```python
from build123d import *

# Parameters (mm, degrees)
F1_DEPTH = 31.75
F3_DEPTH = 31.75
F4_R     = 6.111063
F5_DEPTH = 31.75
F7_DEPTH = 12.7
F9_DEPTH = 25.4


with BuildPart() as f1:
    # F0 (on Front) → F1 (new body)
    with BuildSketch(Plane.XZ):
        Polygon((-42.020088, 46.490617), (-67.420088, 46.490617), (-67.420088, 21.090617), (-3.613756, 21.090617), (-3.613756, 33.790617), (-41.713756, 33.790617), align=None)
    extrude(amount=F1_DEPTH)

    # F2 (on face) → F3 (join)
    with BuildSketch(Plane.XZ.offset(31.75)):
        with BuildLine():
            Line((-67.420088, 46.490617), (-42.020088, 46.490617))
            ThreePointArc((-42.020088, 46.490617), (-54.720088, 59.190617), (-67.420088, 46.490617))
        make_face()
    extrude(amount=-F3_DEPTH)

    # F4 (on face) → F5 (cut)
    with BuildSketch(Plane.XZ.offset(31.75)):
        with Locations((-54.720088, 46.490617)):
            Circle(F4_R)
    extrude(amount=-F5_DEPTH, mode=Mode.SUBTRACT)

    # F6 (on face) → F7 (join)
    with BuildSketch(Plane.XY.offset(33.790617)):
        with BuildLine():
            Line((-3.613756, 0), (-3.613756, -31.75))
            ThreePointArc((-3.613756, -31.75), (12.261244, -15.875), (-3.613756, 0))
        make_face()
    extrude(amount=-F7_DEPTH)

    # F8 (on face) → F9 (cut)
    with BuildSketch(Plane.XY.offset(33.790617)):
        with BuildLine():
            Line((-9.963756, -6.35), (-29.013756, -6.35))
            ThreePointArc((-29.013756, -6.35), (-35.363756, -12.7), (-29.013756, -19.05))
            Line((-29.013756, -19.05), (-9.963756, -19.05))
            ThreePointArc((-9.963756, -19.05), (-3.613756, -12.7), (-9.963756, -6.35))
        make_face()
    extrude(amount=-F9_DEPTH, mode=Mode.SUBTRACT)


solid = f1.part
```
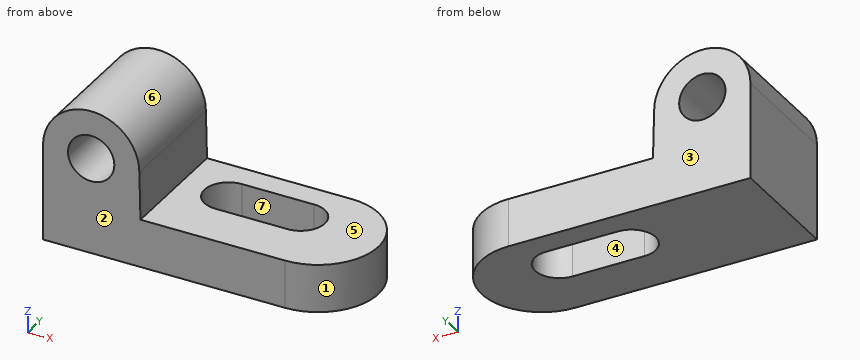
The model under review builds one solid part; all positions refer to its coordinate system, in mm. Face numbers are marked on the shaded views. A direction names the side the tool comes from. Give positions to 0.01 mm unless a question says otherwise; leave off trailing zeros. Write each loop counter-clockwise with the first axis right and the second up, starting at its lowest first coordinate (ties: lowest second). Pieces come first, ordered by that corner, then holes. Notation, with made-up numbers: M 11,-14.5 L 43,-14.5 A19 cw 43,3.5 Z; hole C 47.5,-36 d4. An arc over 180 degrees is marked long. Write item = value, one per line. Start each with the question number.
Q1. For line 1 (Z direction, x = -1.5, y = -1); line 2 (X direction, y = -7.5, z = 46.5); line 3 (Z direction, x = -51.5, y = -1), list the stretches that pass through material, from the lowest coordinate up.
Q2. Mouldability with a two-part tool opening along Y and no side actions: class the marked faces 1, 2, 3 and 4 as released by +Y, released by -Y, zero draft, split by the parting line, or undercut.
Q3. We need section B-B (z = 31.5). State the section outline as (x, y) points (3 decimals).
Q4. Machinability: for the marked faces 5, 6 and 7, which of the approach directions +Z, -Z, +X, -X, +Y, -Y give a long, thin tool a straight path to every point of the face, cutting with its end or side? Answer none if there is none.
Q5. We need section C-C (x = -57). State the section outline as (y, z) points, plus the area to 3 significant figures.
Q6. We need section D-D (y = -3). State the section outline as (x, z) points.
Q7. Clearance check with flat-ended pins moving along their axes: pin 1 (10 mm diameter, centred on x = -38, z = 49.5, fed in from +Y); pin 2 (1 mm diameter, centred on x = -42.5, y = -16.5, fed in from +Z); pin 3 (5 mm diameter, centred on x = -34.5, y = -5.5, fed in from +Z); pin 4 (4 mm diameter, centred on y = -25, z = 54, fed in from -X). State where each tip first meets the part, or that it passes through.
Q8. We need section A-A (y = -12.5). State the section outline as (x, z) points.
Result set:
q1.line_1 = 21.09 to 33.79
q1.line_2 = -67.42 to -60.83, -48.61 to -42.02
q1.line_3 = 21.09 to 41.3, 51.68 to 58.78
q2.face_1 = split by the parting line
q2.face_2 = released by -Y
q2.face_3 = released by +Y
q2.face_4 = undercut
q3.outline = M -67.42,-31.75 L -3.614,-31.75 A15.875 ccw -3.614,0 L -67.42,0 Z; hole M -29.014,-19.05 L -9.964,-19.05 A6.35 ccw -9.964,-6.35 L -29.014,-6.35 A6.35 ccw Z
q4.face_5 = +Z, +X, +Y, -Y
q4.face_6 = +Z, +Y, -Y
q4.face_7 = +Z, -Z
q5.outline = M -31.75,21.09 L 0,21.09 L 0,40.82 L -31.75,40.82 Z; M -31.75,52.16 L 0,52.16 L 0,58.98 L -31.75,58.98 Z
q5.area = 843 mm2
q6.outline = M -67.42,21.09 L 5.67,21.09 L 5.67,33.79 L -41.71,33.79 L -42.02,46.49 A12.7 ccw -67.42,46.49 Z; hole C -54.72,46.49 d12.22
q7.pin_1 = 0
q7.pin_2 = 51.38
q7.pin_3 = 33.79
q7.pin_4 = -66.16
q8.outline = M -67.42,21.09 L -35.36,21.09 L -35.36,33.79 L -41.71,33.79 L -42.02,46.49 A12.7 ccw -67.42,46.49 Z; M -3.62,21.09 L 11.9,21.09 L 11.9,33.79 L -3.62,33.79 Z; hole C -54.72,46.49 d12.22
